Work out the finished part from the listing and answer in its coordinate system (mm). A direction names the side the tool comes from. Coordinates: 2 decimals unless noted, no trailing zeros. Order: outer loops, then holes, each group sorted by start corner. A loop starts at its lowest first (then second) coordinate and runs counter-clockwise, first axis right, second up. Notation, with made-up numbers: M 37,44 L 56,44 A28 ccw 56,66 Z; hole C 53,9 d1. An arc over 180 degrees is marked long. Answer in a Markdown table with one row per item. Add a question column.
Item 1: The part is cut by section D-D (y = -46). Write down the section's boundary in (x, z).
Item 2: The part is cut by section C-C (z = 25.5). Write down the section's boundary in (x, y).
Item 3: The mould has two halves that part along Y. Classify faces 3 (the face through (71.637, 71.389, 19.261)), 4 (the face through (72.2, 1, 18)), 5 (the face through (-0.8, -74.2, 2)): released by +Y, released by -Y, zero draft, split by the parting line, or undercut.
Item 4: The part is cut by section A-A (y = 39). Write down the section's boundary in (x, z).
Item 5: Flat-ended cylindrical pins translate along their axes: pin 1 Ø10 at (x, y) = (11, 49.5) entering from +Z; pin 2 Ø0.6 at (y, z) = (59, 37) entering from +X; pin 3 Ø2 at (y, z) = (59.5, 37) entering from -X; pin 4 Ø1 at (x, z) = (43.5, 37) entering from +Y. Find the tip coordinate at first contact, or state that the pin passes through.
Item 6: The part is cut by section B-B (x = 45). State how many separate pieces and enclosed holes the cut face has, then the cut area to 3 significant figures.
Item 7: Which of the six approach directions +Z, -Z, +X, -X, +Y, -Y give full straight-line access (tool end or side, diameter ignored) to faces 1 (the face through (71.389, -71.637, 19.261)), 2 (the face through (-68.78, 68.59, 17.8))?
Item 8: Consider line 1 (X direction, y = 27.5, z = 22); line 2 (Y direction, x = 15, z = 37.3). Determine where each line is inside the solid, lowest interval first. Write a range as from..to.
from build123d import *

# Parameters (mm, degrees)
SKETCH_W        = 152.4
SKETCH_H        = 152.4
PAD_DEPTH       = 38.1
FILLET_R        = 16
CHAMFER_SIZE    = 4
SKETCH001_R     = 12
SKETCH001_W     = 24
SKETCH001_H     = 6
POCKET_DEPTH    = 38.101
POCKET_FACE9_R  = 12
POCKET_FACE9_W  = 6
POCKET_FACE9_H  = 24
POCKET001_DEPTH = 36.1


with BuildPart() as part:
    # Sketch → Pad (new body)
    with BuildSketch(Plane.XY):
        Rectangle(SKETCH_W, SKETCH_H)
    extrude(amount=PAD_DEPTH)

    # Fillet
    fillet_edges = [part.edges().sort_by_distance(p)[0] for p in [
        (-76.2, 76.2, 19.05),
        (-76.2, -76.2, 19.05),
        (76.2, -76.2, 19.05),
        (76.2, 76.2, 19.05),
    ]]
    fillet(fillet_edges, radius=FILLET_R)

    # Chamfer
    chamfer_edges = [part.edges().sort_by_distance(p)[0] for p in [
        (0, -76.2, 0),
        (0, -76.2, 38.1),
    ]]
    chamfer(chamfer_edges, length=CHAMFER_SIZE)

    # Sketch001 (on Face11 of Chamfer) → Pocket (cut, through all)
    with BuildSketch(Plane.XY.offset(38.1)):
        with Locations((-45, -51)):
            Circle(SKETCH001_R)
        with Locations((-45, -21)):
            Circle(SKETCH001_R)
        with Locations((-45, 9)):
            Circle(SKETCH001_R)
        with Locations((-45, 39)):
            Circle(SKETCH001_R)
        with Locations((-15, -51)):
            Circle(SKETCH001_R)
        with Locations((-15, -21)):
            Circle(SKETCH001_R)
        with Locations((-15, 9)):
            Circle(SKETCH001_R)
        with Locations((-15, 39)):
            Circle(SKETCH001_R)
        with Locations((15, -51)):
            Circle(SKETCH001_R)
        with Locations((15, -21)):
            Circle(SKETCH001_R)
        with Locations((15, 9)):
            Circle(SKETCH001_R)
        with Locations((15, 39)):
            Circle(SKETCH001_R)
        with Locations((45, -51)):
            Circle(SKETCH001_R)
        with Locations((45, -21)):
            Circle(SKETCH001_R)
        with Locations((45, 9)):
            Circle(SKETCH001_R)
        with Locations((45, 39)):
            Circle(SKETCH001_R)
        with Locations((-45, 60)):
            Rectangle(SKETCH001_W, SKETCH001_H)
        with Locations((-15, 60)):
            Rectangle(SKETCH001_W, SKETCH001_H)
        with Locations((15, 60)):
            Rectangle(SKETCH001_W, SKETCH001_H)
        with Locations((45, 60)):
            Rectangle(SKETCH001_W, SKETCH001_H)
    extrude(amount=-POCKET_DEPTH, mode=Mode.SUBTRACT)

    # Pocket Face9 → Pocket001 (cut)
    with BuildSketch(Plane(origin=(0, 0.686829, 0), x_dir=(0, -1, 0), z_dir=(0, 0, -1))):
        with BuildLine():
            Line((72.886829, -60.2), (72.886829, 60.2))
            ThreePointArc((72.886829, 60.2), (69.37211, 68.685281), (60.886829, 72.2))
            Line((60.886829, 72.2), (-59.513171, 72.2))
            ThreePointArc((-59.513171, 72.2), (-67.998453, 68.685281), (-71.513171, 60.2))
            Line((-71.513171, 60.2), (-71.513171, -60.2))
            ThreePointArc((-71.513171, -60.2), (-67.998453, -68.685281), (-59.513171, -72.2))
            Line((-59.513171, -72.2), (60.886829, -72.2))
            ThreePointArc((60.886829, -72.2), (69.37211, -68.685281), (72.886829, -60.2))
        make_face()
        with Locations((-38.313171, 45)):
            Circle(POCKET_FACE9_R, mode=Mode.SUBTRACT)
        with Locations((-8.313171, 45)):
            Circle(POCKET_FACE9_R, mode=Mode.SUBTRACT)
        with Locations((-8.313171, 15)):
            Circle(POCKET_FACE9_R, mode=Mode.SUBTRACT)
        with Locations((-38.313171, 15)):
            Circle(POCKET_FACE9_R, mode=Mode.SUBTRACT)
        with Locations((-38.313171, -15)):
            Circle(POCKET_FACE9_R, mode=Mode.SUBTRACT)
        with Locations((21.686829, 45)):
            Circle(POCKET_FACE9_R, mode=Mode.SUBTRACT)
        with Locations((21.686829, -45)):
            Circle(POCKET_FACE9_R, mode=Mode.SUBTRACT)
        with Locations((-8.313171, -45)):
            Circle(POCKET_FACE9_R, mode=Mode.SUBTRACT)
        with Locations((21.686829, -15)):
            Circle(POCKET_FACE9_R, mode=Mode.SUBTRACT)
        with Locations((-8.313171, -15)):
            Circle(POCKET_FACE9_R, mode=Mode.SUBTRACT)
        with Locations((21.686829, 15)):
            Circle(POCKET_FACE9_R, mode=Mode.SUBTRACT)
        with Locations((-38.313171, -45)):
            Circle(POCKET_FACE9_R, mode=Mode.SUBTRACT)
        with Locations((-59.313171, 45)):
            Rectangle(POCKET_FACE9_W, POCKET_FACE9_H, mode=Mode.SUBTRACT)
        with Locations((-59.313171, 15)):
            Rectangle(POCKET_FACE9_W, POCKET_FACE9_H, mode=Mode.SUBTRACT)
        with Locations((-59.313171, -15)):
            Rectangle(POCKET_FACE9_W, POCKET_FACE9_H, mode=Mode.SUBTRACT)
        with Locations((-59.313171, -45)):
            Rectangle(POCKET_FACE9_W, POCKET_FACE9_H, mode=Mode.SUBTRACT)
        with Locations((51.686829, 15)):
            Circle(POCKET_FACE9_R, mode=Mode.SUBTRACT)
        with Locations((51.686829, -15)):
            Circle(POCKET_FACE9_R, mode=Mode.SUBTRACT)
        with Locations((51.686829, -45)):
            Circle(POCKET_FACE9_R, mode=Mode.SUBTRACT)
        with Locations((51.686829, 45)):
            Circle(POCKET_FACE9_R, mode=Mode.SUBTRACT)
    extrude(amount=-POCKET001_DEPTH, mode=Mode.SUBTRACT)


solid = part.part
Reply:
| question | item | result |
|---|---|---|
| 1 | outline | M -76.2,4 L -72.2,0 L -72.2,36.1 L -55.91,36.1 L -55.91,38.1 L -72.2,38.1 L -76.2,34.1 Z; M -34.09,36.1 L -25.91,36.1 L -25.91,38.1 L -34.09,38.1 Z; M -4.09,36.1 L 4.09,36.1 L 4.09,38.1 L -4.09,38.1 Z; M 25.91,36.1 L 34.09,36.1 L 34.09,38.1 L 25.91,38.1 Z; M 55.91,36.1 L 72.2,36.1 L 72.2,0 L 76.2,4 L 76.2,34.1 L 72.2,38.1 L 55.91,38.1 Z |
| 2 | outline | M -76.2,-60.2 A16 ccw -60.2,-76.2 L 60.2,-76.2 A16 ccw 76.2,-60.2 L 76.2,60.2 A16 ccw 60.2,76.2 L -60.2,76.2 A16 ccw -76.2,60.2 Z; hole M -72.2,-60.2 A12 ccw -60.2,-72.2 L 60.2,-72.2 A12 ccw 72.2,-60.2 L 72.2,60.2 A12 ccw 60.2,72.2 L -60.2,72.2 A12 ccw -72.2,60.2 Z |
| 3 | face 3 | released by +Y |
| 3 | face 4 | undercut |
| 3 | face 5 | released by -Y |
| 4 | outline | M -76.2,4 L -72.2,0 L -72.2,36.1 L -57,36.1 L -57,38.1 L -72.2,38.1 L -76.2,34.1 Z; M -33,36.1 L -27,36.1 L -27,38.1 L -33,38.1 Z; M -3,36.1 L 3,36.1 L 3,38.1 L -3,38.1 Z; M 27,36.1 L 33,36.1 L 33,38.1 L 27,38.1 Z; M 57,36.1 L 72.2,36.1 L 72.2,0 L 76.2,4 L 76.2,34.1 L 72.2,38.1 L 57,38.1 Z |
| 5 | pin 1 | stops at z = 38.1 |
| 5 | pin 2 | stops at x = 73.6 |
| 5 | pin 3 | stops at x = -74.3 |
| 5 | pin 4 | stops at y = 73.8 |
| 6 | separate pieces | 6 |
| 6 | enclosed holes | 0 |
| 6 | area | 358 mm2 |
| 7 | face 1 | +Z, -Z, +X, -Y |
| 7 | face 2 | -Z |
| 8 | line 1 | x = -76.2..-72.2, 72.2..76.2 |
| 8 | line 2 | y = -73..-63, -39..-33, -9..-3, 21..27, 51..57, 63..73 |
